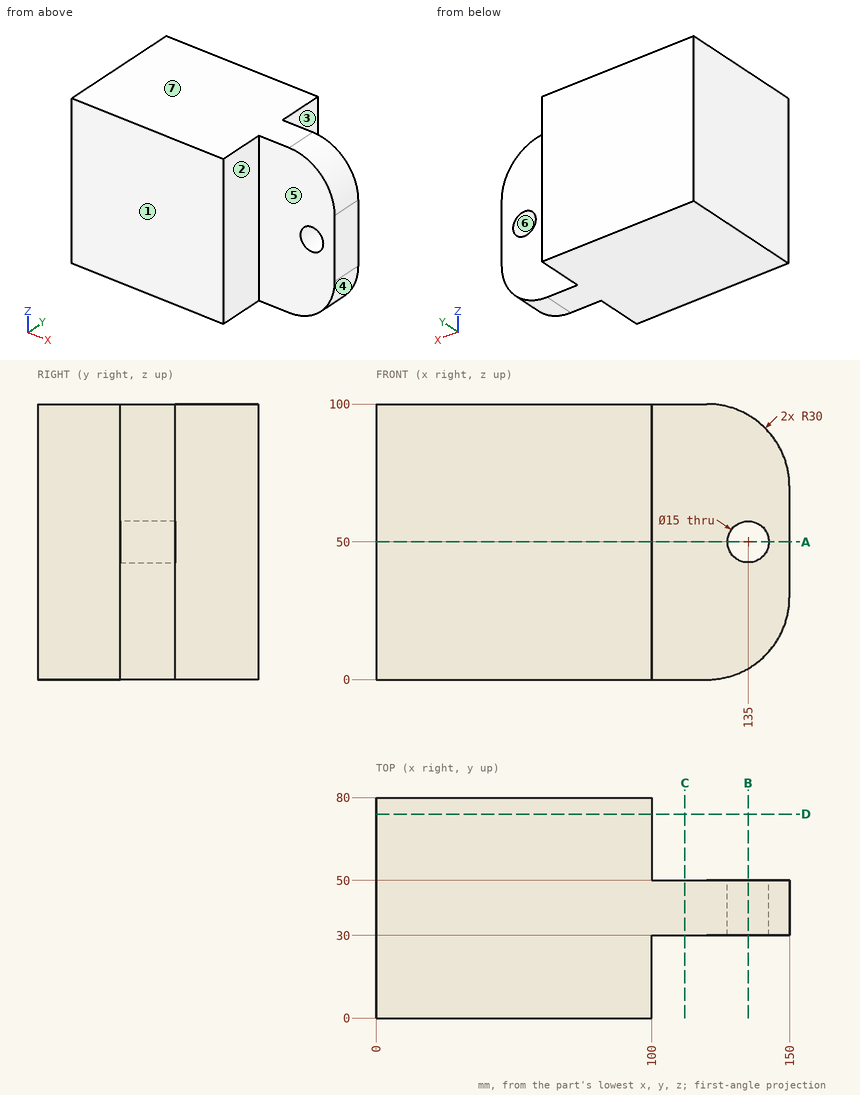
Design review of the part shown in the three views and the two pictorial views. Dimensions are in mm from the part's minimum x, y and z. A direction names the side the tool comes from. Coordinates: 2 decimals unless noted, no trailing zeros. Loops run counter-clockwise (first coordinate to the right, second up) from the corner with the lowest first, then second, coordinate; pieces in that order, holes last. Notation, with made-up numbers: M 46.5,87.25 L 88.5,87.25 A18 cw 88.5,122.25 Z; hole C 54,-25.5 d8. An arc over 180 degrees is marked long. One line per question, with ' | ' between items.
(1) Wall thickness on probe 1 along X at (y, z) = (40, 50); probe 2 along X at (y, z) = (26, 52); probe 3 along Y at (x, z) = (125.5, 39.5): over which ranges is each line inside the solid? List them lowest first.
Filled in:
probe 1: x = 0 to 127.5, 142.5 to 150 | probe 2: x = 0 to 100 | probe 3: y = 30 to 50
(2) We need section A-A (z = 50). Give the boundary of the cut face in (x, y).
Filled in:
outline: M 0,0 L 100,0 L 100,30 L 127.5,30 L 127.5,50 L 100,50 L 100,80 L 0,80 Z; M 142.5,30 L 150,30 L 150,50 L 142.5,50 Z
(3) We need section D-D (y = 74). Give the boundary of the cut face in (x, z), and give its area (3 significant figures).
Filled in:
outline: M 0,0 L 100,0 L 100,100 L 0,100 Z | area: 10,000 mm^2
(4) We need section C-C (x = 112). Give the boundary of the cut face in (y, z).
Filled in:
outline: M 30,0 L 50,0 L 50,100 L 30,100 Z
(5) For pin 1 Ø1 at (x, z) = (130, 63.5) entering from -Y; pin 2 Ø1.5 at (y, z) = (28.5, 71) entering from +X, all flat-tipped, find the tip position at first contact; note any pin that passes through.
Filled in:
pin 1: stops at y = 30 | pin 2: stops at x = 100
(6) We need section B-B (x = 135). Give the boundary of the cut face in (y, z), and give its area (3 significant figures).
Filled in:
outline: M 30,4.02 L 50,4.02 L 50,42.5 L 30,42.5 Z; M 30,57.5 L 50,57.5 L 50,95.98 L 30,95.98 Z | area: 1,540 mm^2
(7) Machinability: for the marked faces 1, 2 and 3, which of the approach directions +Z, -Z, +X, -X, +Y, -Y give a long, thin tool a straight path to every point of the face, cutting with its end or side? Answer none if there is none.
Filled in:
face 1: +Z, -Z, +X, -X, -Y | face 2: +Z, -Z, +X, -Y | face 3: +Z, -Z, +X, +Y
(8) Draft analysis for pull direction Z (two halves, no side actions). For the marked faces 4, 5, 6 and 7, state which applies: released by +Z, released by -Z, zero draft, split by the parting line, or undercut.
Filled in:
face 4: released by -Z | face 5: zero draft | face 6: undercut | face 7: released by +Z
